The listing builds one solid part. Answer for the finished solid, in the listing's coordinates (mm). A direction names the side the tool comes from. Give positions to 0.01 mm unless a question says otherwise; leave off trailing zeros. Write each loop counter-clockwise with the first axis right and the second up, starting at its lowest first coordinate (ties: lowest second). Pieces come first, ordered by that corner, then holes. Notation, with made-up numbers: (-36, 21) -> (16, 21) arc R12 ccw to (16, 34) -> close; hole circle Ø2 at (31.5, 27.5). An arc over 180 degrees is marked (long way). Put each result on its own line as item: value. Start each with the question number.
1) A cutting plane is placed at A-A (x = -2.5). Write down the section's boundary in (y, z), then the cut area to 3 significant figures.
2) For a pull along Y with two mould halves and no side action, classify faces 1 (the cylindrical face through (-49.9, 32.62, 1.57)), 2 (the flat face through (-25, 1.549, 2)), 3 (the flat face through (-50.8, 16, 2)), 4 (the flat face through (0, 0, 2)) as released by +Y, released by -Y, zero draft, split by the parting line, or undercut.
3) A cutting plane is placed at D-D (x = 82). Write down the section's boundary in (y, z).
4) Find the intervals of material crossed by line 1 along Y through (x, z) = (44.45, 1.25); line 2 along Y through (x, z) = (76.2, 2.3); line 3 along X through (y, z) = (0.5, 2.2), in increasing order. Write a range as from..to.
5) For faces 5 (the flat face through (-50.8, -8, 2)), 6 (the flat face through (-26, -1.549, 2)), determine the directions among +Z, -Z, +X, -X, +Y, -Y from which every point of the face is accessible in a straight line to the end or side of a thin tool.
6) A cutting plane is placed at C-C (y = 41.5). Write down the section's boundary in (x, z).
7) A flat-ended cylindrical pin translates along its axis: pin 1 Ø1.7 at (x, y) = (76.2, 0) entering from -Z. Find the tip coordinate at first contact, or state that the pin passes through.
8) A cutting plane is placed at B-B (z = 1.8). Write down the section's boundary in (x, y).
from build123d import *

# Parameters (mm, degrees)
BOSS_EXTRUDE1_DEPTH = 3.0988
SKETCH3_R           = 1.0795
SKETCH3_R_2         = 9.3726
BOSS_EXTRUDE2_DEPTH = 3.0988
FILLET1_R           = 5.08


with BuildPart() as part:
    # Sketch2 → Boss-Extrude1 (new body)
    with BuildSketch(Plane.XY):
        Polygon((-50.8, 1.5494), (-50.8, 7.8994), (50.8, 7.8994), (50.8, -7.8994), (-50.8, -7.8994), (-50.8, -1.5494), (0, -1.5494), (0, 1.5494), align=None)
    extrude(amount=BOSS_EXTRUDE1_DEPTH)

    # Sketch3 → Boss-Extrude2 (add)
    with BuildSketch(Plane.XY):
        with BuildLine():
            Line((50.8, -7.8994), (-50.8, -7.8994))
            Line((-50.8, -7.8994), (-50.8, -20.5994))
            Line((-50.8, -20.5994), (101.6, -20.5994))
            Line((101.6, -20.5994), (101.6, 33.2994))
            Line((101.6, 33.2994), (54.782161872, 63.523702231))
            ThreePointArc((54.782161872, 63.523702231), (46.597523005, 66.447615713), (37.96588061, 65.431577828))
            Line((37.96588061, 65.431577828), (-50.8, 33.2994))
            Line((-50.8, 33.2994), (-50.8, 7.8994))
            Line((-50.8, 7.8994), (50.8, 7.8994))
            Line((50.8, 7.8994), (50.8, -7.8994))
        make_face()
        with Locations((76.2, 0)):
            Circle(SKETCH3_R, mode=Mode.SUBTRACT)
        with Locations((44.45, 47.519048812)):
            Circle(SKETCH3_R_2, mode=Mode.SUBTRACT)
    extrude(amount=BOSS_EXTRUDE2_DEPTH)

    # Fillet1
    fillet1_edges = [part.edges().sort_by_distance(p)[0] for p in [
        (101.6, 33.2994, 1.5494),
        (-50.8, 33.2994, 1.5494),
        (-50.8, -20.5994, 1.5494),
        (101.6, -20.5994, 1.5494),
    ]]
    fillet(fillet1_edges, radius=FILLET1_R)


solid = part.part
Reply:
1. outline: (-20.6, 0) -> (-1.55, 0) -> (-1.55, 3.1) -> (-20.6, 3.1) -> close; (1.55, 0) -> (50.78, 0) -> (50.78, 3.1) -> (1.55, 3.1) -> close
1. area: 212 mm2
2. face 1: released by +Y
2. face 2: undercut
2. face 3: zero draft
2. face 4: undercut
3. outline: (-20.6, 0) -> (45.95, 0) -> (45.95, 3.1) -> (-20.6, 3.1) -> close
4. line 1: y = -20.6..38.15, 56.89..66.57
4. line 2: y = -20.6..-1.08, 1.08..49.7
4. line 3: x = 0..75.24, 77.16..101.6
5. face 5: +Z, -Z, -X, +Y, -Y
5. face 6: +Z, -Z, -X
6. outline: (-28.15, 0) -> (37.27, 0) -> (37.27, 3.1) -> (-28.15, 3.1) -> close; (51.63, 0) -> (88.9, 0) -> (88.9, 3.1) -> (51.63, 3.1) -> close
7. pin 1: passes through
8. outline: (-50.8, -15.52) arc R5.08 ccw to (-45.72, -20.6) -> (96.52, -20.6) arc R5.08 ccw to (101.6, -15.52) -> (101.6, 30.53) arc R5.08 ccw to (99.28, 34.8) -> (54.78, 63.52) arc R19.05 ccw to (37.97, 65.43) -> (-47.45, 34.51) arc R5.08 ccw to (-50.8, 29.74) -> (-50.8, 1.55) -> (0, 1.55) -> (0, -1.55) -> (-50.8, -1.55) -> close; hole circle Ø18.75 at (44.45, 47.52); hole circle Ø2.16 at (76.2, 0)
